Design review of the part built by this model. Coordinates are the model's own, in mm. Coordinates: 2 decimals unless noted, no trailing zeros. Write each loop counter-clockwise with the first axis right and the second up, starting at its lowest first coordinate (ties: lowest second). Pieces come first, ordered by that corner, then holes. Notation, with made-up numbers: (-5, 80.25) - (28, 80.25) arc R29 ccw to (28, 103.25) - close; hole circle Ø11 at (2, 84). An arc over 180 degrees is marked (long way). Use a Markdown table: item, result.
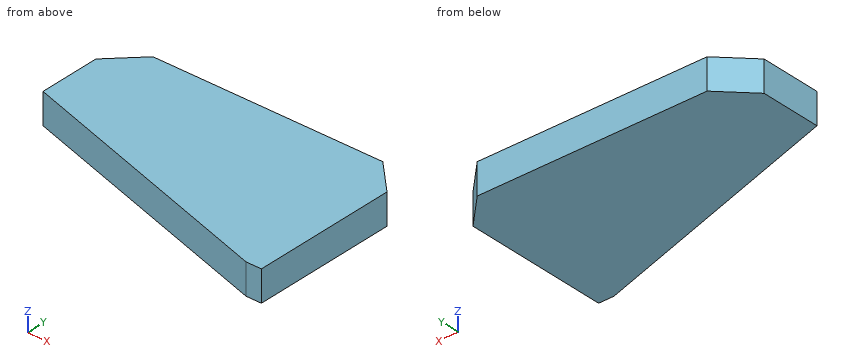
from build123d import *

# Parameters (mm, degrees)
SM_START               = -5
SM_BASE_FLANGE_1_DEPTH = 10
CHAMFER_1_SIZE         = 10


# Read off the part's stored shape, not the designer's step: Базовая кромка1
with BuildPart() as part:
    # Базовая кромка1 outline → Базовая кромка1 (new body)
    with BuildSketch(Plane.XY.offset(SM_START)):
        Polygon((0, 0), (-95, 0), (-95, -30), (-5, -57.5), (0, -57.5), align=None)
    extrude(amount=SM_BASE_FLANGE_1_DEPTH)

    # Фаска1
    chamfer_1_edges = [part.edges().sort_by_distance(p)[0] for p in [
        (-95, 0, 0),
        (0, 0, 0),
    ]]
    chamfer(chamfer_1_edges, length=CHAMFER_1_SIZE)


solid = part.part
(1) Take a section at C-C on x = -20.5. Write out the cut boundary in (y, z), and give its area (3 significant figures).
Determined:
| item | result |
|---|---|
| outline | (-52.76, -5) - (0, -5) - (0, 5) - (-52.76, 5) - close |
| area | 528 mm2 |
(2) For pin 1 (4 mm diameter, centred on x = -78, z = -2.5, fed in from -Y); pin 2 (3 mm diameter, centred on x = -85.5, z = 2, fed in from -Y); pin 3 (1.5 mm diameter, centred on x = -50, z = 1.5, fed in from -Y), all flat-tipped, find the tip position at first contact; note any pin that passes through.
Determined:
| item | result |
|---|---|
| pin 1 | y = -35.81 |
| pin 2 | y = -33.36 |
| pin 3 | y = -43.98 |
(3) Take a section at B-B on y = -4. Write out the cut boundary in (x, z), and give its area (3 significant figures).
Determined:
| item | result |
|---|---|
| outline | (-89, -5) - (-6, -5) - (-6, 5) - (-89, 5) - close |
| area | 830 mm2 |
(4) Take a section at A-A on z = 0. Write out the cut boundary in (x, y), and give its area (4 significant figures).
Determined:
| item | result |
|---|---|
| outline | (-95, -30) - (-5, -57.5) - (0, -57.5) - (0, -10) - (-10, 0) - (-85, 0) - (-95, -10) - close |
| area | 4,125 mm2 |
(5) For L1, parallel to Y at x = -5, z = 2; L2, parallel to Y at x = -68, z = 4.25; L3, parallel to X at y = -5, z = 1.75, list the stretches that pass through material, from the lowest coordinate up. Write a range as from..to.
Determined:
| item | result |
|---|---|
| L1 | -57.5..-5 |
| L2 | -38.25..0 |
| L3 | -90..-5 |
